For this review, use the dimensioned drawing (mm, ordinates from the lowest corner) and the shaded views. Coordinates: 2 decimals unless noted, no trailing zeros. Order: outer loops, then holes, each group sorted by start corner. A loop starts at its lowest first (then second) coordinate and runs counter-clockwise, first axis right, second up. Notation, with made-up numbers: M 63.25,88 L 83.25,88 A7 ccw 83.25,93 Z; hole C 49.5,55.25 d3. An arc over 180 degrees is marked long. Answer as CSV lines item,"result". Start each with the question number.
Q1. For P1, Ø4, axis at x = 34.49, z = 13, coming from the -Y side; P2, Ø0.9, axis at x = 77.5, y = 1, coming from the +Z side, all flat-tipped, find the tip position at first contact; note any pin that passes through.
Q2. Consider section B-B on y = 1.45. Write out the cut boundary in (x, z) (1 decimal), and give its area (3 significant figures).
Q3. Consider section C-C on z = 44.5. Write out the cut boundary in (x, y), and give its area (3 significant figures).
Q4. Consider section A-A on z = 13. Write out the cut boundary in (x, y) (1 decimal).
Q5. Wall thickness on L1, parallel to X at y = 0.4, z = 13 (1 decimal); L2, parallel to X at y = 0.5, z = 25 (1 decimal); L3, parallel to X at y = 0.95, z = 33.5 (1 decimal): over which ranges is each line inside the solid? List them lowest first. Write a range as [from, to].
Q6. Consider section D-D on x = 74.5. Write out the cut boundary in (y, z).
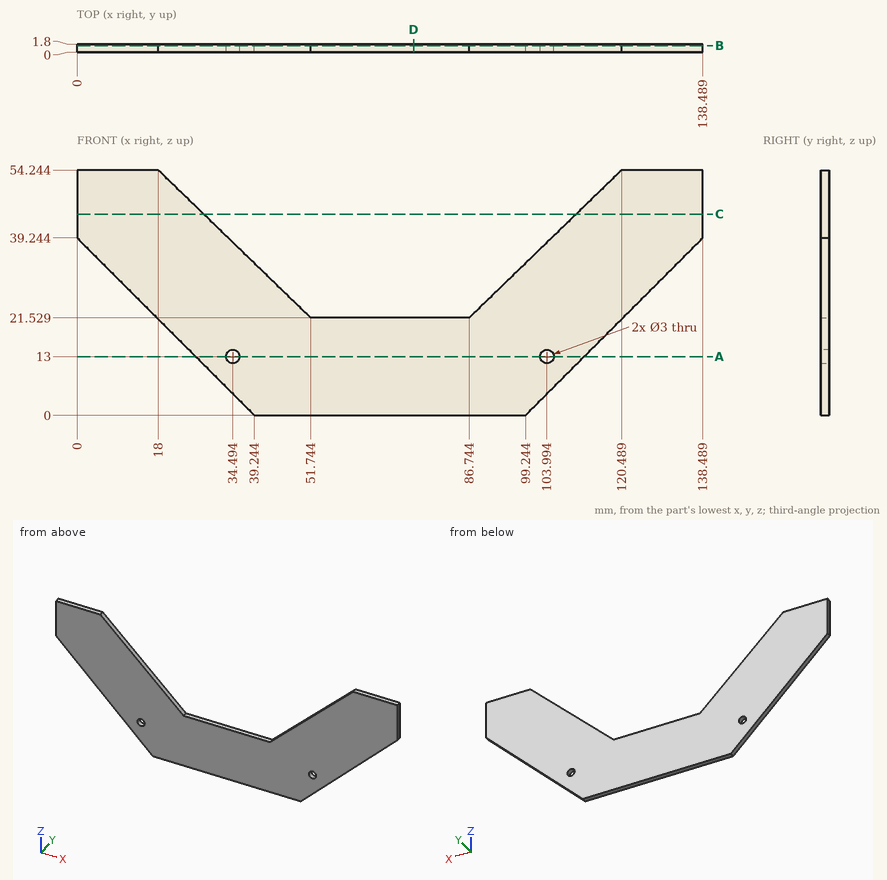
Evaluation:
1,P1,"stops at y = 0"
1,P2,"stops at z = 21.53"
2,outline,"M 0,39.2 L 39.2,0 L 99.2,0 L 138.5,39.2 L 138.5,54.2 L 120.5,54.2 L 86.7,21.5 L 51.7,21.5 L 18,54.2 L 0,54.2 Z; hole C 34.5,13 d3; hole C 104,13 d3"
2,area,"3,710 mm²"
3,outline,"M 0,0 L 28.05,0 L 28.05,1.8 L 0,1.8 Z; M 110.44,0 L 138.49,0 L 138.49,1.8 L 110.44,1.8 Z"
3,area,"101 mm²"
4,outline,"M 26.2,0 L 33,0 L 33,1.8 L 26.2,1.8 Z; M 36,0 L 102.5,0 L 102.5,1.8 L 36,1.8 Z; M 105.5,0 L 112.2,0 L 112.2,1.8 L 105.5,1.8 Z"
5,L1,"x = [26.2, 33], [36, 102.5], [105.5, 112.2]"
5,L2,"x = [14.2, 48.2], [90.3, 124.2]"
5,L3,"x = [5.7, 39.4], [99.1, 132.7]"
6,outline,"M 0,0 L 1.8,0 L 1.8,21.53 L 0,21.53 Z"
